The listing builds one solid part. Answer for the finished solid, in the listing's coordinates (mm). A direction names the side the tool comes from. Round coordinates to 2 decimals unless told otherwise and drop trailing zeros. Order: outer loops, then holes, each group sorted by start corner. A loop starts at its lowest first (then second) coordinate and runs counter-clockwise, first axis right, second up. Notation, with made-up numbers: (9, -19.5) -> (29, -19.5) arc R19 ccw to (29, 2.5) -> close; hole circle Ø8 at (-14, 56). An arc over 180 degrees is marked (long way). Answer in a Markdown table with one row per item. Add a question column.
```python
from build123d import *

# Parameters (mm, degrees)
ESQUISSE1_R               = 1.5
T_LE_DE_BASE_PLI_E1_DEPTH = 4


# Sheet-metal steps are written as plain solids
with BuildPart() as part:
    # Esquisse1 → Tôle de base pliée1 (new body)
    with BuildSketch(Plane.XY):
        with BuildLine():
            Line((-17, -12.348242597), (-17, -235))
            ThreePointArc((-17, -235), (0, -252), (17, -235))
            Line((17, -235), (17, -12.348242597))
            Line((17, -12.348242597), (11.921461884, 3.758822494))
            ThreePointArc((11.921461884, 3.758822494), (0, 12.5), (-11.921461884, 3.758822494))
            Line((-11.921461884, 3.758822494), (-17, -12.348242597))
        make_face()
        Circle(ESQUISSE1_R, mode=Mode.SUBTRACT)
        with Locations((0, -150)):
            Circle(ESQUISSE1_R, mode=Mode.SUBTRACT)
        with BuildLine():
            Line((-5, -235), (-5, -219))
            ThreePointArc((-5, -219), (0, -214), (5, -219))
            Line((5, -219), (5, -235))
            ThreePointArc((5, -235), (0, -240), (-5, -235))
        make_face(mode=Mode.SUBTRACT)
    extrude(amount=-T_LE_DE_BASE_PLI_E1_DEPTH)


solid = part.part
```
Item 1: Find the intervals of material crossed by probe 1 along Y at (x, z) = (0, -3.1); probe 2 along Y at (x, z) = (-0.5, -2.6); probe 3 along X at (y, z) = (-231, -0.9), in increasing order. Write a range as [from, to].
Item 2: For a pull along Y with two mould halves and no side action, classify faces 3 (the face through (0, -214, -2)), 4 (the face through (0, -252, -2)), 5 (the face through (0, -118, -4)) as released by +Y, released by -Y, zero draft, split by the parting line, or undercut.
Item 3: The part is cut by section C-C, the plane x = -9. Give the vertices of the cut face in (y, z), and give its area (3 significant figures).
Item 4: The part is cut by section B-B, the plane y = -223. Give the vertices of the cut face in (x, z).
Item 5: A tool of negligible diameter and unlimited length cuts with its end or side. For faces 1 (the face through (0, -240, -2)), 2 (the face through (0.2, 12.5, -2)), from which of +Z, -Z, +X, -X, +Y, -Y can it reach the whole face along a straight path? Write none if from no direction.
Item 6: The part is cut by section A-A, the plane z = -1.9. Give the vertices of the cut face in (x, y).
Item 7: The part is cut by section D-D, the plane y = -8.5. Give the vertices of the cut face in (x, z), and give its area (3 significant figures).
Resolved:
| question | item | result |
|---|---|---|
| 1 | probe 1 | [-252, -240], [-214, -151.5], [-148.5, -1.5], [1.5, 12.5] |
| 1 | probe 2 | [-251.99, -239.97], [-214.03, -151.41], [-148.59, -1.41], [1.41, 12.49] |
| 1 | probe 3 | [-17, -5], [5, 17] |
| 2 | face 3 | undercut |
| 2 | face 4 | released by -Y |
| 2 | face 5 | zero draft |
| 3 | outline | (-249.42, -4) -> (8.67, -4) -> (8.67, 0) -> (-249.42, 0) -> close |
| 3 | area | 1,030 mm2 |
| 4 | outline | (-17, -4) -> (-5, -4) -> (-5, 0) -> (-17, 0) -> close; (5, -4) -> (17, -4) -> (17, 0) -> (5, 0) -> close |
| 5 | face 1 | +Z, -Z |
| 5 | face 2 | +Z, -Z, +Y |
| 6 | outline | (-17, -235) arc R17 ccw to (17, -235) -> (17, -12.35) -> (11.92, 3.76) arc R12.5 ccw to (-11.92, 3.76) -> (-17, -12.35) -> close; hole (-5, -235) arc R5 ccw to (5, -235) -> (5, -219) arc R5 ccw to (-5, -219) -> close; hole circle Ø3 at (0, -150); hole circle Ø3 at (0, 0) |
| 7 | outline | (-15.79, -4) -> (15.79, -4) -> (15.79, 0) -> (-15.79, 0) -> close |
| 7 | area | 126 mm2 |
